For this review, take the finished solid that the model builds, in its own axes (mm). A direction names the side the tool comes from. Coordinates: 2 decimals unless noted, no trailing zeros. Write each loop counter-clockwise with the first axis right and the second up, starting at its lowest first coordinate (ties: lowest second). Pieces come first, ordered by that corner, then holes. Notation, with made-up numbers: (-35.75, 86) -> (-25.75, 86) arc R18 cw to (-25.75, 100) -> close; hole circle Ø9 at (-16, 43). An arc over 180 degrees is marked (long way). One line per item, written item: value. Start each with the question number.
1) For probe 1 along Z at (x, y) = (12.7, 48.75) (1 decimal); probe 2 along Y at (x, z) = (2.2, 25.4) (3 decimals); probe 3 along X at (y, z) = (20, 12.5) (3 decimals), list the stretches that pass through material, from the lowest coordinate up. Write a range as from..to.
2) Add section A-A (x = 12.7). State the section outline as (y, z) points (1 decimal).
3) Add section D-D (z = 5). State the section outline as (x, y) points (3 decimals), and give its area (3 significant figures).
4) Add section C-C (z = 25.5). State the section outline as (x, y) points (3 decimals), and give its area (3 significant figures).
5) Mouldability with a two-part tool opening along Y and no side actions: class faces 3 (the flat face through (17, 48, 17)), 4 (the cylindrical face through (1.61, 10.768, 12.045)), 5 (the cylindrical face through (1.61, 11.48, 22.47)), 6 (the flat face through (2, 33, 0)) as released by +Y, released by -Y, zero draft, split by the parting line, or undercut.
6) Machinability: for faces 1 (the flat face through (25.4, 50, 17)), 2 (the flat face through (3.175, 24, 17)), which of the approach directions +Z, -Z, +X, -X, +Y, -Y give a long, thin tool a straight path to every point of the face, cutting with its end or side? Answer none if there is none.
7) For pin 1 Ø4 at (y, z) = (35.5, 4) entering from +X (3 decimals); pin 2 Ø6 at (x, z) = (11, 13) entering from -Y, all flat-tipped, find the tip position at first contact; note any pin that passes through.
8) Add section B-B (y = 12.7). State the section outline as (x, z) points (3 decimals), and give its area (3 significant figures).
from build123d import *

# Parameters (mm, degrees)
BOSS_EXTRUDE1_DEPTH = 34.925
SKETCH2_R           = 3.175
CUT_EXTRUDE1_DEPTH  = 4.175
SKETCH3_R           = 2.5
CUT_EXTRUDE2_DEPTH  = 52.175


with BuildPart() as part:
    # Sketch1 → Boss-Extrude1 (new body)
    with BuildSketch(Plane.XY):
        Polygon((0, 0), (3.175, 0), (3.175, 48), (25.4, 48), (25.4, 51.175), (0, 51.175), align=None)
    extrude(amount=BOSS_EXTRUDE1_DEPTH)

    # Sketch2 → Cut-Extrude1 (cut, through all)
    with BuildSketch(Plane(origin=(3.175, 0, 0), x_dir=(0, 0, -1), z_dir=(1, 0, 0))):
        with Locations((-25.4, 12.7)):
            Circle(SKETCH2_R)
        with Locations((-9.525, 12.7)):
            Circle(SKETCH2_R)
    extrude(amount=-CUT_EXTRUDE1_DEPTH, mode=Mode.SUBTRACT)

    # Sketch3 → Cut-Extrude2 (cut, through all)
    with BuildSketch(Plane(origin=(0, 51.175, 0), x_dir=(1, 0, 0), z_dir=(0, 1, 0))):
        with Locations((12.7, -17.4625)):
            Circle(SKETCH3_R)
    extrude(amount=-CUT_EXTRUDE2_DEPTH, mode=Mode.SUBTRACT)


solid = part.part
Numbers:
1. probe 1: 0..15, 20..34.9
1. probe 2: 0..9.525, 15.875..51.175
1. probe 3: 0..3.175
2. outline: (48, 0) -> (51.2, 0) -> (51.2, 15) -> (48, 15) -> close; (48, 20) -> (51.2, 20) -> (51.2, 34.9) -> (48, 34.9) -> close
3. outline: (0, 0) -> (3.175, 0) -> (3.175, 48) -> (25.4, 48) -> (25.4, 51.175) -> (0, 51.175) -> close
3. area: 233 mm²
4. outline: (0, 0) -> (3.175, 0) -> (3.175, 9.527) -> (0, 9.527) -> close; (0, 15.873) -> (3.175, 15.873) -> (3.175, 48) -> (25.4, 48) -> (25.4, 51.175) -> (0, 51.175) -> close
4. area: 213 mm²
5. face 3: released by -Y
5. face 4: undercut
5. face 5: undercut
5. face 6: zero draft
6. face 1: +Z, -Z, +X, +Y, -Y
6. face 2: +Z, -Z, +X, -Y
7. pin 1: x = 3.175
7. pin 2: y = 48
8. outline: (0, 0) -> (3.175, 0) -> (3.175, 6.35) -> (0, 6.35) -> close; (0, 12.7) -> (3.175, 12.7) -> (3.175, 22.225) -> (0, 22.225) -> close; (0, 28.575) -> (3.175, 28.575) -> (3.175, 34.925) -> (0, 34.925) -> close
8. area: 70.6 mm²
